Part model, mm, in its own coordinate system. Face numbers are marked on the shaded views. A direction names the side the tool comes from. Round coordinates to 2 decimals unless told otherwise and drop trailing zeros. Write each loop counter-clockwise with the first axis right and the second up, starting at its lowest first coordinate (ties: lowest second). Pieces come first, ordered by that corner, then holes. Notation, with made-up numbers: M 36,28.5 L 77,28.5 A28 ccw 77,58.5 Z; hole C 35,70.5 d3. An arc over 180 degrees is marked long. Use a Markdown table: item, result. Add a question column.
1) Slice it at C-C on y = -0.75. Write the cut outline in (x, z), plus the area to 3 significant figures.
2) Slice it at B-B on z = 18. Write the cut outline in (x, y), plus the area to 3 significant figures.
3) Slice it at A-A on x = 0. Write the cut outline in (y, z), plus the area to 3 significant figures.
4) Two-plate mould, pull along Z, no slides. Class the marked faces 1, 2 and 3: released by +Z, released by -Z, zero draft, split by the parting line, or undercut.
5) Slice it at D-D on x = -6. Write the cut outline in (y, z).
6) Wall check: probe 1 along Z at (x, y) = (0, -10.3); probe 2 along Z at (x, y) = (5, 3.5); probe 3 along Y at (x, z) = (0.25, 18.5). Give the ranges that are in metal, low to high.
7) Drop flat-ended pins along their axis: P1, Ø5, axis at x = 4, y = -3, coming from the -Z side; P2, Ø2, axis at x = 3, z = 4, coming from the -Y side; P3, Ø1.5, axis at x = -1, z = 24, coming from the +Y side. Give the stop position or say it passes through.
8) Which spindle directions (+Z, -Z, +X, -X, +Y, -Y) get a long thin tool onto all of the face, cutting with end or side? Do the marked faces 4 and 5. Say none if no direction does.
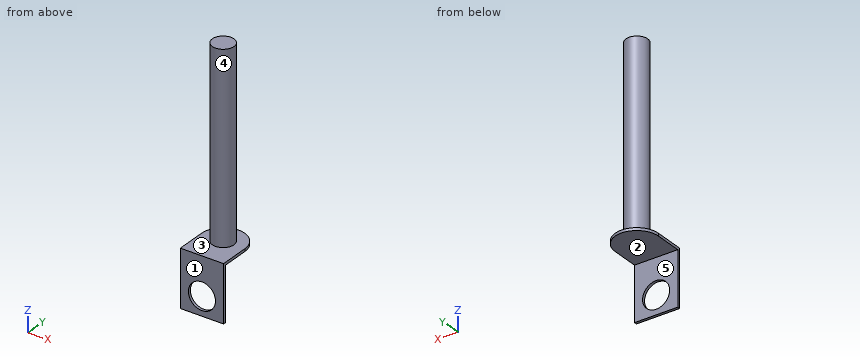
```python
from build123d import *

# Parameters (mm, degrees)
SKETCH1_R           = 4
BOSS_EXTRUDE1_DEPTH = 69
BOSS_EXTRUDE2_DEPTH = 1
SKETCH3_W           = 16
SKETCH3_H           = 20
BOSS_EXTRUDE3_DEPTH = 1
SKETCH4_W           = 16
SKETCH4_H           = 1
BOSS_EXTRUDE4_DEPTH = 1
SKETCH5_R           = 5
CUT_EXTRUDE1_DEPTH  = 1


with BuildPart() as part:
    # Sketch1 → Boss-Extrude1 (new body)
    with BuildSketch(Plane.XY):
        Circle(SKETCH1_R)
    extrude(amount=BOSS_EXTRUDE1_DEPTH)

    # Sketch2 → Boss-Extrude2 (add)
    with BuildSketch(Plane(origin=(0, 0, 0), x_dir=(-1, 0, 0), z_dir=(0, 0, -1))):
        with BuildLine():
            Line((-8, 0), (-8, -10))
            Line((-8, -10), (8, -10))
            Line((8, -10), (8, 0))
            ThreePointArc((8, 0), (0, 8), (-8, 0))
        make_face()
    extrude(amount=BOSS_EXTRUDE2_DEPTH)



with BuildPart() as body_2:
    # Sketch3 → Boss-Extrude3 (new body)
    with BuildSketch(Plane.XZ.offset(10)):
        with Locations((0, -11)):
            Rectangle(SKETCH3_W, SKETCH3_H)
    extrude(amount=BOSS_EXTRUDE3_DEPTH)


with BuildPart() as part_1:
    add(part.part)

    add(body_2.part)  # Boss-Extrude4 merges body 2
    # Sketch4 → Boss-Extrude4 (add)
    with BuildSketch(Plane.XY.offset(-1)):
        with Locations((0, -10.5)):
            Rectangle(SKETCH4_W, SKETCH4_H)
    extrude(amount=BOSS_EXTRUDE4_DEPTH)

    # Sketch5 → Cut-Extrude1 (cut)
    with BuildSketch(Plane(origin=(0, -10, 0), x_dir=(1, 0, 0), z_dir=(0, 1, 0))):
        with Locations((0, 14.046188681)):
            Circle(SKETCH5_R)
    extrude(amount=-CUT_EXTRUDE1_DEPTH, mode=Mode.SUBTRACT)


solid = part_1.part
```
Entries:
| question | item | result |
|---|---|---|
| 1 | outline | M -8,-1 L 8,-1 L 8,0 L 3.93,0 L 3.93,69 L -3.93,69 L -3.93,0 L -8,0 Z |
| 1 | area | 558 mm^2 |
| 2 | outline | C 0,0 d8 |
| 2 | area | 50.3 mm^2 |
| 3 | outline | M -11,-21 L -10,-21 L -10,-19.05 L -11,-19.05 Z; M -11,-9.05 L -10,-9.05 L -10,-1 L 8,-1 L 8,0 L 4,0 L 4,69 L -4,69 L -4,0 L -11,0 Z |
| 3 | area | 581 mm^2 |
| 4 | face 1 | zero draft |
| 4 | face 2 | released by -Z |
| 4 | face 3 | released by +Z |
| 5 | outline | M -11,-21 L -10,-21 L -10,-1 L 5.29,-1 L 5.29,0 L -11,0 Z |
| 6 | probe 1 | z = -21 to -19.05, -9.05 to 0 |
| 6 | probe 2 | z = -1 to 0 |
| 6 | probe 3 | y = -3.99 to 3.99 |
| 7 | P1 | stops at z = -1 |
| 7 | P2 | stops at y = -3.46 |
| 7 | P3 | stops at y = 3.99 |
| 8 | face 4 | +Z |
| 8 | face 5 | -Z, +X, -X, +Y |
